from build123d import *

# Parameters (mm, degrees)
BOX007_W              = 11
BOX007_H              = 7
BOX007_DEPTH          = 10
FILLET_R              = 3
ARRAY_COUNT           = 2
ARRAY_ANGLE           = 180
ARRAY_PLACEMENT_ANGLE = 90
CYLINDER004_R         = 3
CYLINDER004_DEPTH     = 30
CYLINDER_R            = 3.5
CYLINDER_DEPTH        = 15
CYLINDER006_R         = 6
CYLINDER006_DEPTH     = 4
CYLINDER005_R         = 6
CYLINDER005_DEPTH     = 4
BOX001_W              = 5
BOX001_H              = 10
BOX001_DEPTH          = 5
BOX002_W              = 20
BOX002_H              = 25
BOX002_DEPTH          = 5
BOX_W                 = 20
BOX_H                 = 5
BOX_DEPTH             = 20


with BuildPart() as array:
    # Box007 → Box007 (new body)
    with BuildSketch(Plane(origin=(10, 5, -5), x_dir=(1, 0, 0), z_dir=(0, 0, 1))):
        with Locations((5.5, 3.5)):
            Rectangle(BOX007_W, BOX007_H)
    extrude(amount=BOX007_DEPTH)


with BuildPart() as array_1:
    # BaseFeature placement: moved
    add(array.part.moved(Location((-10, -5, 5))))

    # Fillet
    fillet_edges = [array_1.edges().sort_by_distance(p)[0] for p in [
        (5.5, 0, 10),
        (5.5, 0, 0),
    ]]
    fillet(fillet_edges, radius=FILLET_R)


with BuildPart() as array_2:
    # Body placement: moved
    add(array_1.part.moved(Location((-5, 5, 0))))

    # Array: Array ×2 about axis
    array_axis = Axis((0, 0, 0), (0, 0, 1))


with BuildPart() as array_3:
    add(array_2.part)
    for i in range(1, ARRAY_COUNT):
        add(array_2.part.rotate(array_axis, i * ARRAY_ANGLE / (ARRAY_COUNT - 1)))


with BuildPart() as array_4:
    # Array placement: moved
    add(array_3.part.moved(Location((0, -3, -5))).rotate(Axis((0, -3, -5), (0, 0, 1)), ARRAY_PLACEMENT_ANGLE))


with BuildPart() as cilindro004:
    # Cylinder004 → Cylinder004 (new body)
    with BuildSketch(Plane(origin=(0, 15, -15), x_dir=(1, 0, 0), z_dir=(0, 0, 1))):
        Circle(CYLINDER004_R)
    extrude(amount=CYLINDER004_DEPTH)


with BuildPart() as cilindro:
    # Cylinder → Cylinder (new body)
    with BuildSketch(Plane.XZ.offset(-5)):
        Circle(CYLINDER_R)
    extrude(amount=CYLINDER_DEPTH)


with BuildPart() as obj1:
    # Cylinder006 → Cylinder006 (new body)
    with BuildSketch(Plane.XY.offset(4.3)):
        Circle(CYLINDER006_R)
    extrude(amount=CYLINDER006_DEPTH)


with BuildPart() as fusion003:
    # Cylinder005 → Cylinder005 (new body)
    with BuildSketch(Plane.XY.offset(-8.3)):
        Circle(CYLINDER005_R)
    extrude(amount=CYLINDER005_DEPTH)

    # Fusion003: union obj1
    add(obj1.part)


with BuildPart() as fusion003_1:
    # Fusion003 placement: moved
    add(fusion003.part.moved(Location((0, 15, 0))))


with BuildPart() as pin0:
    # Box001 → Box001 (new body)
    with BuildSketch(Plane(origin=(-2.5, -10, 5), x_dir=(1, 0, 0), z_dir=(0, 0, 1))):
        with Locations((2.5, 5)):
            Rectangle(BOX001_W, BOX001_H)
    extrude(amount=BOX001_DEPTH)


with BuildPart() as pin001:
    # Clone base: copy of pin0
    add(pin0.part)


with BuildPart() as pin001_1:
    # Clone placement: moved
    add(pin001.part.moved(Location((0, 0, -15))))


with BuildPart() as pared1:
    # Box002 → Box002 (new body)
    with BuildSketch(Plane(origin=(-10, 0, 5), x_dir=(1, 0, 0), z_dir=(0, 0, 1))):
        with Locations((10, 12.5)):
            Rectangle(BOX002_W, BOX002_H)
    extrude(amount=BOX002_DEPTH)


with BuildPart() as pared002:
    # Clone001 base: copy of pared1
    add(pared1.part)


with BuildPart() as pared002_1:
    # Clone001 placement: moved
    add(pared002.part.moved(Location((0, 0, -15))))


with BuildPart() as cut003:
    # Box → Box (new body)
    with BuildSketch(Plane(origin=(-10, -5, -10), x_dir=(1, 0, 0), z_dir=(0, 0, 1))):
        with Locations((10, 2.5)):
            Rectangle(BOX_W, BOX_H)
    extrude(amount=BOX_DEPTH)

    # Fusion: union pin0, pin001, pared1, pared002
    add(pin0.part)
    add(pin001_1.part)
    add(pared1.part)
    add(pared002_1.part)

    # Fusion004: union Fusion003
    add(fusion003_1.part)

    # Cut001: cut Cilindro
    add(cilindro.part, mode=Mode.SUBTRACT)

    # Cut002: cut Cilindro004
    add(cilindro004.part, mode=Mode.SUBTRACT)

    # Cut003: cut Array
    add(array_4.part, mode=Mode.SUBTRACT)


solid = cut003.part
Model file for the job. Use its own axes, mm. A direction names the side the tool comes from. Round coordinates to 2 decimals unless told otherwise and drop trailing zeros. Order: outer loops, then holes, each group sorted by start corner. A loop starts at its lowest first (then second) coordinate and runs counter-clockwise, first axis right, second up.
(1) Band-saw the part on B-B (x = 0). Give the number of separate pieces and of enclosed holes in the cut face, then the cut area to 3 significant figures.
(2) Pull direction Y, two halves, no side cores. Call faces 5 (the face through (1.7, 0, -3.4)), 6 (the face through (0, 8, -10)), 7 (the face through (0, 25, 7)): released by +Y, released by -Y, zero draft, split by the parting line, or undercut.
(3) Band-saw the part on D-D (y = 6). List the corners of the cut face in (x, z).
(4) 3-axis set-ups, long thin cutter, end or side, ignore diameter. For faces 1 (the face through (5.86, -2.54, -4.1)), 2 (the face through (2.5, -8, 7)), 3 (the face through (-2.5, -8, 7)), 4 (the face through (0, -7, 5)): which of +Z, -Z, +X, -X, +Y, -Y reach the whole face in a straight line?
(5) Band-saw the part on C-C (z = 0). List the corners of the cut face in (x, y), then the cut area to 3 significant figures.
(6) Band-saw the part on A-A (y = 15). List the corners of the cut face in (x, z), then the cut area to 3 significant figures.
(7) Drill centre lines: line 1 (Z direction, x = -0.75, y = 1); line 2 (Y direction, x = 0, z = -8.2); line 3 (X direction, y = 15, z = 5.9). Where is each one in solid material? Low to high.
(8) Pin check, flat tips, straight feed: pin 1 (5 mm diameter, centred on x = 6.5, z = 2.5, fed in from -Y); pin 2 (5.5 mm diameter, centred on x = 0, z = 0, fed in from -Y); pin 3 (2.5 mm diameter, centred on y = -7.5, z = 8.5, fed in from +X); pin 4 (2.5 mm diameter, centred on y = -8.5, z = 7.5, fed in from -X). Stop position of each tip, or through.
Verdict:
1. separate pieces: 4
1. enclosed holes: 0
1. area: 313 mm2
2. face 5: undercut
2. face 6: zero draft
2. face 7: released by +Y
3. outline: (-10, -10) - (10, -10) - (10, -5) - (-10, -5) - close; (-10, 5) - (10, 5) - (10, 10) - (-10, 10) - close
4. face 1: +X, +Y, -Y
4. face 2: +Z, -Z, +X, -Y
4. face 3: +Z, -Z, -X, -Y
4. face 4: +X, -X, -Y
5. outline: (-5, -5) - (-3.5, -5) - (-3.5, 0) - (-5, 0) - close; (3.5, -5) - (5, -5) - (5, 0) - (3.5, 0) - close
5. area: 15.0 mm2
6. outline: (-10, -10) - (-3, -10) - (-3, -4.3) - (-6, -4.3) - (-6, -5) - (-10, -5) - close; (-10, 5) - (-6, 5) - (-6, 4.3) - (-3, 4.3) - (-3, 10) - (-10, 10) - close; (3, -10) - (10, -10) - (10, -5) - (6, -5) - (6, -4.3) - (3, -4.3) - close; (3, 4.3) - (6, 4.3) - (6, 5) - (10, 5) - (10, 10) - (3, 10) - close
6. area: 148 mm2
7. line 1: z = -10 to -5, 5 to 10
7. line 2: y = -10 to 12, 18 to 25
7. line 3: x = -10 to -3, 3 to 10
8. pin 1: stops at y = -5
8. pin 2: passes through
8. pin 3: stops at x = 2.5
8. pin 4: stops at x = -2.5
